Verification items for this drawing (mm, ordinates from the low corner). A direction names the side the tool comes from. Round coordinates to 2 decimals unless told otherwise and drop trailing zeros. Loops run counter-clockwise (first coordinate to the right, second up) from the corner with the lowest first, then second, coordinate; pieces in that order, holes last. Notation, with made-up numbers: (-7.75, 71) - (36.25, 71) arc R18 ccw to (36.25, 98) - close; hole circle Ø5 at (11.5, -7). An arc over 180 degrees is marked (long way). Put each result on its own line as item: value.
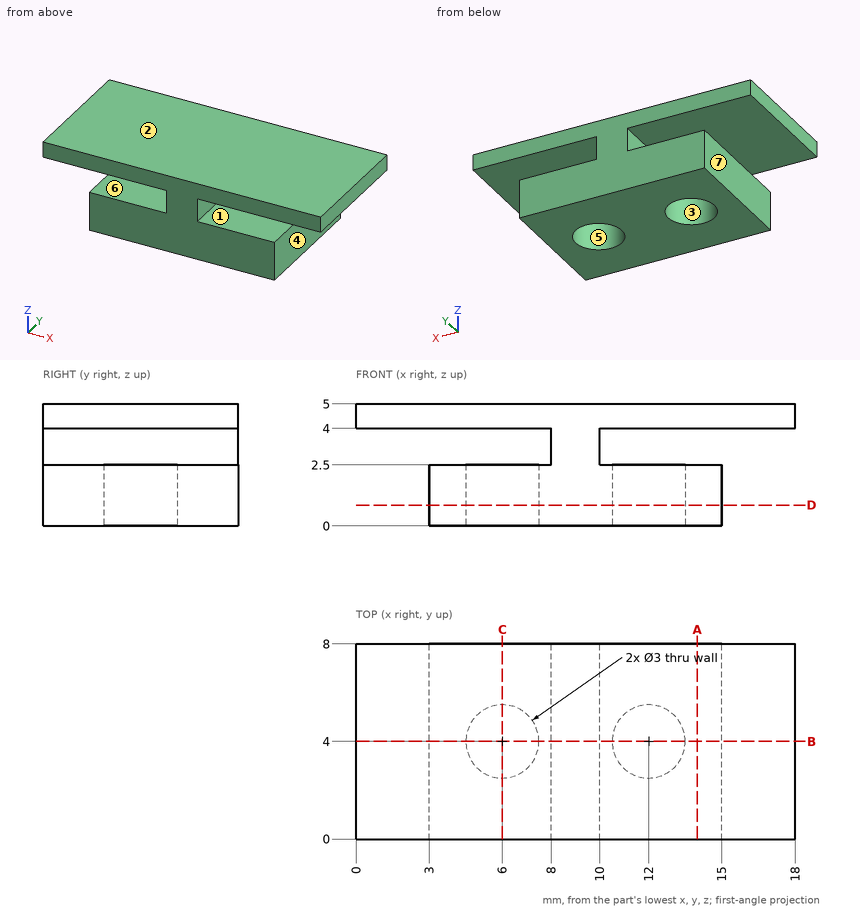
Item 1: Tool access check on the marked faces 4, 5, 6 and 7. Record the directions out of +Z, -Z, +X, -X, +Y, -Y that give a thin tool (end or side, any length) a straight path to the whole face; none if there is none.
Filled sheet:
face 4: -Z, +X, +Y, -Y
face 5: -Z
face 6: -X, +Y, -Y
face 7: -Z, -X, +Y, -Y
Item 2: Section check B-B on y = 4. Enter the section's corners in (x, z), then the cut area to 3 significant figures.
Filled sheet:
outline: (0, 4) - (8, 4) - (8, 2.5) - (7.5, 2.5) - (7.5, 0) - (10.5, 0) - (10.5, 2.5) - (10, 2.5) - (10, 4) - (18, 4) - (18, 5) - (0, 5) - close; (3, 0) - (4.5, 0) - (4.5, 2.5) - (3, 2.5) - close; (13.5, 0) - (15, 0) - (15, 2.5) - (13.5, 2.5) - close
area: 36.0 mm²
Item 3: Section check C-C on x = 6. Enter the section's corners in (y, z), then the cut area to 3 significant figures.
Filled sheet:
outline: (0, 0) - (2.5, 0) - (2.5, 2.5) - (0, 2.5) - close; (0, 4) - (8, 4) - (8, 5) - (0, 5) - close; (5.5, 0) - (8, 0) - (8, 2.5) - (5.5, 2.5) - close
area: 20.5 mm²
Item 4: Release check for a two-part mould opening along Z. For the marked faces 1, 2 and 3 record: +Z half, -Z half, draft (parallel to the pull), parting line (faces both ways), or undercut.
Filled sheet:
face 1: undercut
face 2: +Z half
face 3: draft
Item 5: Go/stop test with flat-tipped pins: pin 1 (3 mm diameter, centred on y = 5, z = 1, fed in from +X); pin 2 (1.6 mm diameter, centred on y = 5, z = 3, fed in from -X). Record where each tip stops, or that it passes through.
Filled sheet:
pin 1: x = 15
pin 2: x = 3
Item 6: Section check A-A on x = 14. Enter the section's corners in (y, z), then the cut area to 3 significant figures.
Filled sheet:
outline: (0, 0) - (8, 0) - (8, 2.5) - (0, 2.5) - close; (0, 4) - (8, 4) - (8, 5) - (0, 5) - close
area: 28.0 mm²
Item 7: Thickness scan on line 1 (Z direction, x = 3.5, y = 3.25); line 2 (Y direction, x = 6, z = 1.05); line 3 (X direction, y = 6.5, z = 3.05). Record the ranges inside material, lowest first. Write a range as from..to.
Filled sheet:
line 1: 0..2.5, 4..5
line 2: 0..2.5, 5.5..8
line 3: 8..10
Item 8: Section check D-D on z = 0.85. Enter the section's corners in (x, y), then the cut area to 3 significant figures.
Filled sheet:
outline: (3, 0) - (15, 0) - (15, 8) - (3, 8) - close; hole circle Ø3 at (6, 4); hole circle Ø3 at (12, 4)
area: 81.9 mm²
